Part model, mm, in its own coordinate system. A direction names the side the tool comes from. Round coordinates to 2 decimals unless told otherwise and drop trailing zeros. Order: outer loops, then holes, each group sorted by start corner. A loop starts at its lowest first (then second) coordinate and runs counter-clockwise, first axis right, second up. Notation, with made-up numbers: (28, 3) -> (82, 3) arc R29 ccw to (82, 27) -> close; hole circle Ø2 at (-33, 63). An arc over 180 degrees is marked (long way). Return JSON: item names as keys, results as strings. Group by question number.
Autodesk Inventor part; units mm, degrees
ref_plane "Work Plane1" through (30.1625, 0, 0) normal (0, 0, -1) x (1, 0, 0)
ref_plane "YZ Plane" through (0, 0, 0) normal (1, 0, 0) x (0, 1, 0)
ref_plane "XZ Plane" through (0, 0, 0) normal (0, 1, 0) x (-1, 0, 0)
sketch "Skizze1" plane through (0, 0, 0) normal (0, 0, 1) x (1, 0, 0)
  line L0 (-1.8, 0) -> (5, 0)
  line L1 (5, 0) -> (5, 1.5)
  line L2 (5, 1.5) -> (1, 1.5)
  line L3 (1, 1.5) -> (0.6932, 1.3467)
  line L4 (0.6932, 1.3467) -> (0, 1.3467)
  line L5 (0, 1.3467) -> (0, 2.8)
  line L6 (-3.16, 0) -> (6.36, 0)
  line L7 (0, -0.56) -> (0, 3.36)
  line L8 (-1.8, 0) -> (-1.8, 2.6425)
  line L9 (0, 2.8) -> (-1.8, 2.6425)
  line L10 (1, 1.5) -> (0, 1.5) construction
  dimension "d0" = 5
  dimension "d1" = 4
  dimension "d2" = 0.3068
  dimension "d3" = 1.8
  dimension "d4" = 3
  dimension "d5" = 2.6935
  dimension "d9" = 5.6
  dimension "d10" = 5
revolve "Körper" add sketch "Skizze1" angle 360 about axis through (-1.8, 0, 0) along (1, 0, 0)
sketch "Skizze2" plane through (-1.8, 0, 0) normal (-1, 0, 0) x (0, 0, 1)
  circle A0 centre (0, 0) radius 2.8
  line L0 (0, 0) -> (0, 2.6425)
  line L1 (-2.8, 0.4) -> (2.8, 0.4)
  line L2 (2.8, 0.4) -> (2.8, -0.4)
  line L3 (2.8, -0.4) -> (-2.8, -0.4)
  line L4 (-2.8, -0.4) -> (-2.8, 0.4)
  line L5 (-2.8, 0) -> (2.8, 0) construction
  line L6 (0, 0.4) -> (0, -0.4) construction
  dimension "d11" = 0.8
  dimension "d12" = 5.6
fillet "Rundung1" radius 0.9 1 edges at (-1.8, -2.6425, 0)
extrude "Loch" cut sketch "Skizze2" against normal blind 0.7 contours A0 L3 L1 | L2 L3 A0 | A0 L1 L2 | A0 L4 L1 | L3 L4 A0
thread "Gewinde"
ref_plane "Work Plane1" through (30.1625, 0, 0) normal (0, 0, -1) x (1, 0, 0)
fillet "Fillet5" radius 0.1 1 edges at (0, -1.3467, 0)
equation "\"d11\" = SBR"
equation "\"d12\" = KOD"
equation "\"d14\" = RR"
equation "\"d19\" = STI"
equation "\"d15\" = GEL"
equation "\"d41\" = R"
equation "\"d0\" = NLG"
equation "\"d1\" = GEL"
equation "\"d3\" = KOH"
equation "\"d4\" = GD"
equation "\"d5\" = BDM"
equation "\"d9\" = KOD"
equation "\"d10\" = KEWI"
equation "\"GD\" = NND"
equation "\"NLG\" = 5"
equation "\"GEL\" = 4"
equation "\"KOD\" = 5.6"
equation "\"KOH\" = 1.8"
equation "\"GAL\" = 0.61345 * PTC"
equation "\"R\" = 0.1"
equation "\"BDM\" = 2.6935"
equation "\"GUL\" = 0.61345 * PTC"
equation "\"RR\" = 0.9"
equation "\"SBR\" = 0.8"
equation "\"STI\" = 0.7"
equation "\"KEWI\" = 5deg"
equation "\"PTC\" = 0.5"
equation "\"THREADDIA\" = 3"
equation "\"TOA\" = 30deg"
equation "\"NND\" = 3"
equation "\"GD1\" = THREADDIA - 1.2269 * PTC"
properties part number "ISO 1580 - M3 x 5" material "Stahl, weich"
(1) Tool access for faces 1 (the cylindrical face through (2.97, -1.5, -0.07)), 2 (the flat face through (-1.8, 1, 0)), 3 (the cylindrical face through (0.39, -1.07, 0.82)): list every direction of +Z, -Z, +X, -X, +Y, -Y with a clear straight run to the whole face (end or side of a thin tool).
(2) Pin check, flat tips, straight feed: P1, Ø1.5, axis at x = 0.5, z = -1, coming from the +Y side; P2, Ø0.8, axis at x = -1.5, z = 0.5, coming from the +Y side; P3, Ø0.6, axis at x = -1.5, z = -1, coming from the -Y side. Stop position of each tip, or through.
(3) Saw through at C-C, the plane x = 0.5. List the corners of the cut face in (y, z), and give its area (3 significant figures).
(4) Saw through at B-B, the plane z = 0. List the corners of the cut face in (x, y).
(5) Mould opens along Y. For faces 4 (the conical face through (-0.7, -2.17, -1.67)), 5 (the flat face through (-1.1, 0, 0)), 6 (the flat face through (0, 1.2, -1.2)) say: pulls with the +Y half, pulls with the -Y half, needs draft (parallel to the pull), parting line crosses it, or undercut.
(6) Saw through at D-D, the plane x = 3.25. List the corners of the cut face in (y, z).
(7) Saw through at A-A, the plane y = 0. List the corners of the cut face in (x, z).
(8) Probe L1, parallel to X at y = 1, z = 1.6; L2, parallel to X at y = -1, z = -2.4; L3, parallel to Z at x = 2.25, y = 0.85. List the from-to ranges inside material, lowest first. Write a range as [from, to].
Results are:
{
 "1": {"face 1": "+X", "face 2": "+Z, -Z, -X, +Y, -Y", "face 3": "none"},
 "2": {"P1": "stops at y = 2.77", "P2": "stops at y = 2.67", "P3": "stops at y = -2.51"},
 "3": {"outline": "circle Ø2.69 at (0, 0)", "area": "5.70 mm^2"},
 "4": {"outline": "(-1.8, -1.82) arc R0.9 ccw to (-0.98, -2.71) -> (0, -2.8) -> (0, -1.45) arc R0.1 cw to (0.1, -1.35) -> (0.69, -1.35) -> (1, -1.5) -> (5, -1.5) -> (5, 1.5) -> (1, 1.5) -> (0.69, 1.35) -> (0.1, 1.35) arc R0.1 cw to (0, 1.45) -> (0, 2.8) -> (-0.98, 2.71) arc R0.9 ccw to (-1.8, 1.82) -> (-1.8, 0.4) -> (-1.1, 0.4) -> (-1.1, -0.4) -> (-1.8, -0.4) -> close"},
 "5": {"face 4": "parting line crosses it", "face 5": "undercut", "face 6": "needs draft"},
 "6": {"outline": "circle Ø3 at (0, 0)"},
 "7": {"outline": "(-1.1, -2.7) arc R0.9 ccw to (-0.98, -2.71) -> (0, -2.8) -> (0, -1.45) arc R0.1 cw to (0.1, -1.35) -> (0.69, -1.35) -> (1, -1.5) -> (5, -1.5) -> (5, 1.5) -> (1, 1.5) -> (0.69, 1.35) -> (0.1, 1.35) arc R0.1 cw to (0, 1.45) -> (0, 2.8) -> (-0.98, 2.71) arc R0.9 ccw to (-1.1, 2.7) -> close"},
 "8": {"L1": "x = [-1.8, 0]", "L2": "x = [-1.35, 0]", "L3": "z = [-1.24, 1.24]"}
}
